Design review of the part built by this model. Coordinates are the model's own, in mm. A direction names the side the tool comes from. Coordinates: 2 decimals unless noted, no trailing zeros. Loops run counter-clockwise (first coordinate to the right, second up) from the corner with the lowest first, then second, coordinate; pieces in that order, holes last. Notation, with made-up numbers: (41.5, 79) -> (49.5, 79) arc R19 ccw to (49.5, 89) -> close; hole circle Ø4 at (65, 65.5). An arc over 180 degrees is marked (long way). Use a Markdown table: item, result. Add a question column.
Q1. For faces 1 (the face through (0, 0, 0)), 2 (the face through (0, -2, 76.2)), 3 (the face through (-0.63, 1, 18.16)), list the 3-axis set-ups (+Z, -Z, +X, -X, +Y, -Y) from which the entire face can be reached by the end or side of a thin tool; tool diameter is ignored.
Q2. Take a section at A-A on x = 0. Write out the cut boundary in (y, z).
Q3. Clearance check with a flat-ended pin moving along its axis: pin 1 Ø1 at (x, z) = (1, 38) entering from -Y. State where the tip first meets the part, or that it passes through.
Q4. Take a section at C-C on z = 30. Write out the cut boundary in (x, y).
Q5. For probe 1 along Y at (x, z) = (0, 24.5); probe 2 along Y at (x, z) = (-0.25, 62.5); probe 3 along Z at (x, y) = (-1.5, -0.25), list the stretches that pass through material, from the lowest coordinate up.
from build123d import *

# Parameters (mm, degrees)
SKETCH1_R           = 3.9497
BOSS_EXTRUDE1_DEPTH = 78.74
CUT_EXTRUDE1_START  = -2.54
SKETCH2_R           = 3.9497
SKETCH2_R_2         = 1.5875
CUT_EXTRUDE1_DEPTH  = 2.54
SKETCH4_R           = 3.9497
SKETCH4_R_2         = 1.1811
CUT_EXTRUDE3_DEPTH  = 36.83
CHAMFER1_SIZE       = 4.064
CHAMFER1_SIZE2      = 2.346351494


with BuildPart() as part:
    # Sketch1 → Boss-Extrude1 (new body)
    with BuildSketch(Plane.XY):
        Circle(SKETCH1_R)
    extrude(amount=BOSS_EXTRUDE1_DEPTH)

    # Sketch2 → Cut-Extrude1 (cut)
    with BuildSketch(Plane.XY.offset(78.74).offset(CUT_EXTRUDE1_START)):
        Circle(SKETCH2_R)
        Circle(SKETCH2_R_2, mode=Mode.SUBTRACT)
    extrude(amount=CUT_EXTRUDE1_DEPTH, mode=Mode.SUBTRACT)

    # Sketch4 → Cut-Extrude3 (cut)
    with BuildSketch(Plane(origin=(0, 0, 0), x_dir=(-1, 0, 0), z_dir=(0, 0, -1))):
        Circle(SKETCH4_R)
        Circle(SKETCH4_R_2, mode=Mode.SUBTRACT)
    extrude(amount=-CUT_EXTRUDE3_DEPTH, mode=Mode.SUBTRACT)

    # Chamfer1
    chamfer1_edges = [part.edges().sort_by_distance(p)[0] for p in [
        (-3.9497, 0, 36.83),
    ]]
    chamfer1_side = [part.faces().sort_by_distance(p)[0] for p in [
        (-3.9497, 0, 56.515),
    ]]
    chamfer(chamfer1_edges, length=CHAMFER1_SIZE, length2=CHAMFER1_SIZE2, reference=chamfer1_side[0])


solid = part.part
Answer list:
| question | item | result |
|---|---|---|
| 1 | face 1 | -Z, +X, -X, +Y, -Y |
| 1 | face 2 | +Z |
| 1 | face 3 | -Z |
| 2 | outline | (-3.95, 40.89) -> (-1.6, 36.83) -> (-1.18, 36.83) -> (-1.18, 0) -> (1.18, 0) -> (1.18, 36.83) -> (1.6, 36.83) -> (3.95, 40.89) -> (3.95, 76.2) -> (1.59, 76.2) -> (1.59, 78.74) -> (-1.59, 78.74) -> (-1.59, 76.2) -> (-3.95, 76.2) -> close |
| 3 | pin 1 | y = -2.42 |
| 4 | outline | circle Ø2.36 at (0, 0) |
| 5 | probe 1 | -1.18 to 1.18 |
| 5 | probe 2 | -3.94 to 3.94 |
| 5 | probe 3 | 36.83 to 78.74 |
